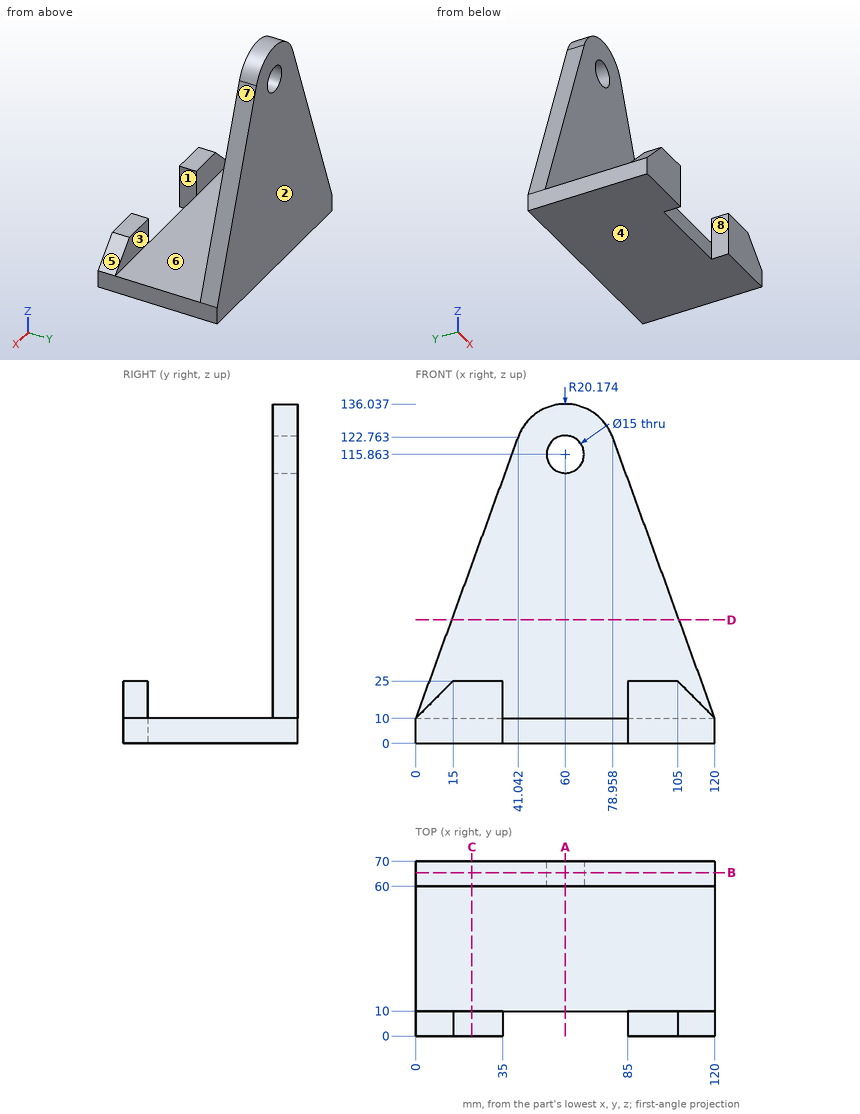
Geometry check sheet. Reference: drawing and pictorial views, mm from the part's lowest x, y, z. A direction names the side the tool comes from. Give positions to 0.01 mm unless a question says otherwise; leave off trailing zeros. Order: outer loops, then holes, each group sorted by start corner. A loop starts at its lowest first (then second) coordinate and runs counter-clockwise, first axis right, second up. Notation, with made-up numbers: M 32,-29 L 59,-29 A36 ccw 59,9 Z; hole C 29,0.25 d7. An arc over 180 degrees is marked long. Use one line per item in the form item = value. Start each with the question number.
Q1. Section check A-A (x = 60). Enter the section's corners in (y, z).
Q2. Access from +Z, -Z, +X, -X, +Y, -Y to the whole of each face (thin tool, end or side, straight path). Record for the marked faces 4, 5, 6, 7 and 8.
Q3. Scan lines: line 1 along Z through (x, y) = (111, 32.5); line 2 along Y through (x, z) = (14, 25.5); line 3 along X through (y, z) = (4, 7.5). Record each from-to range of solid material in increasing order. Write a range as [from, to].
Q4. Section check D-D (z = 49.5). Enter the section's corners in (x, y).
Q5. Go/stop test with flat-tipped pins: pin 1 Ø5 at (x, y) = (91, 7.5) entering from +Z; pin 2 Ø1.5 at (x, z) = (18.5, 25) entering from -Y; pin 3 Ø5 at (x, z) = (52.5, 6) entering from -Y; pin 4 Ø25 at (x, y) = (60.5, 36.5) entering from +Z. Record where each tip stops, or that it passes through.
Q6. Section check B-B (y = 65.5). Enter the section's corners in (x, z) (1 decimal).
Q7. Mould release check, pull along Y, two halves, no side actions. Record for the marked faces 1, 2 and 3: +Y half, -Y half, draft (parallel to the pull), parting line (faces both ways), or undercut.
Q8. Section check C-C (x = 22.5). Enter the section's corners in (y, z).
Evaluation:
q1.outline = M 10,0 L 70,0 L 70,108.36 L 60,108.36 L 60,10 L 10,10 Z; M 60,123.36 L 70,123.36 L 70,136.04 L 60,136.04 Z
q2.face_4 = -Z, +X, -X, +Y, -Y
q2.face_5 = +Z, +X, -Y
q2.face_6 = +Z, +X, -X
q2.face_7 = +Z, +X, +Y, -Y
q2.face_8 = +Z, -Z, -Y
q3.line_1 = [0, 10]
q3.line_2 = [60, 70]
q3.line_3 = [0, 35], [85, 120]
q4.outline = M 14.38,60 L 105.62,60 L 105.62,70 L 14.38,70 Z
q5.pin_1 = 25
q5.pin_2 = 0
q5.pin_3 = 10
q5.pin_4 = 10
q6.outline = M 0,0 L 120,0 L 120,10 L 79,122.8 A20.2 ccw 41,122.8 L 0,10 Z; hole C 60,115.9 d15
q7.face_1 = draft
q7.face_2 = +Y half
q7.face_3 = undercut
q8.outline = M 0,0 L 70,0 L 70,71.82 L 60,71.82 L 60,10 L 10,10 L 10,25 L 0,25 Z
